Print and shaded views of the part. All mm, measured from the part's lowest x, y and z. Round coordinates to 2 decimals unless told otherwise and drop trailing zeros. Loops run counter-clockwise (first coordinate to the right, second up) from the corner with the lowest first, then second, coordinate; pieces in that order, holes last. Notation, with made-up numbers: (8.5, 31) - (14.5, 31) arc R28 cw to (14.5, 52) - close; hole circle Ø5 at (29, 12). An arc over 180 degrees is marked (long way). Use one line per item in the form item = value. Start each with the question number.
Q1. Pin check, flat tips, straight feed: pin 1 (5 mm diameter, centred on x = 70, z = 14.5, fed in from -Y); pin 2 (1.5 mm diameter, centred on y = 2, z = 17, fed in from +X); pin 3 (5 mm diameter, centred on x = 38, y = 8.5, fed in from +Z); pin 4 (1 mm diameter, centred on y = 5, z = 13.5, fed in from +X). Stop position of each tip, or through.
Q2. Saw through at B-B (y = 2). Give the cut face in (x, z).
Q3. Drill centre lines: line 1 (Z direction, x = 134, y = 1); line 2 (Z direction, x = 241.5, y = 1.5); line 3 (X direction, y = 3.5, z = 21.5). Where is each one in solid material? Low to high.
Q4. Saw through at A-A (x = 293). Give the cut face in (y, z).
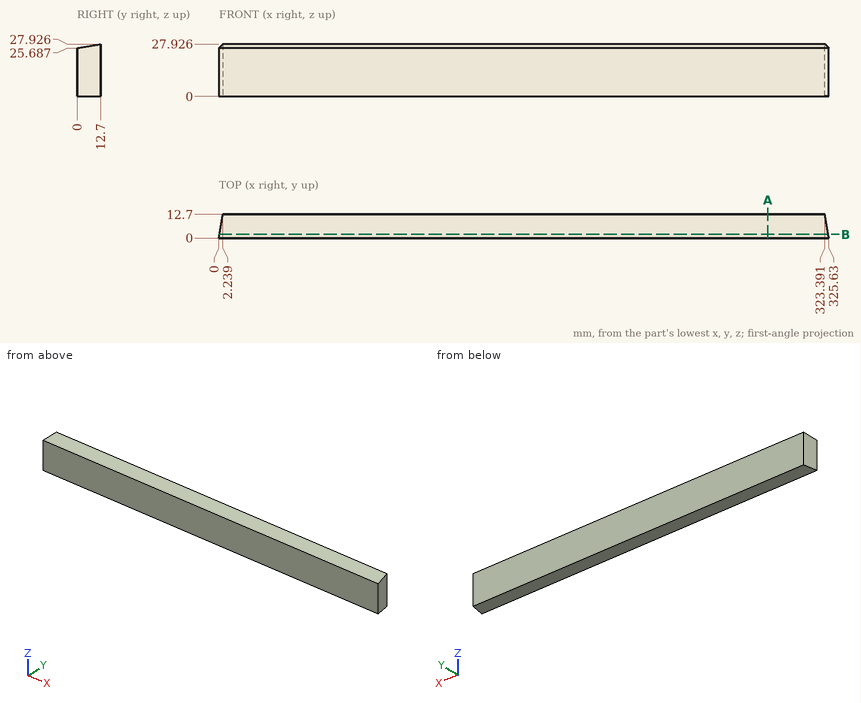
Report:
q1.pin_1 = 0
q1.pin_2 = 325.41
q1.pin_3 = 27.63
q1.pin_4 = 324.84
q2.outline = (0.35, 0) - (325.28, 0) - (325.28, 26.04) - (0.35, 26.04) - close
q3.line_1 = 0 to 25.86
q3.line_2 = 0 to 25.95
q3.line_3 = 0.62 to 325.01
q4.outline = (0, 0) - (12.7, 0) - (12.7, 27.93) - (0, 25.69) - close
